Design review of the part built by this model. Coordinates are the model's own, in mm. Face numbers are marked on the shaded views. A direction names the side the tool comes from. Give positions to 0.01 mm unless a question says otherwise; leave off trailing zeros. Write each loop counter-clockwise with the first axis right and the second up, starting at its lowest first coordinate (ties: lowest second). Pieces come first, ordered by that corner, then holes. Notation, with made-up numbers: (-33.75, -26.5) -> (-7.75, -26.5) arc R24 cw to (-7.75, -6.5) -> close; hole circle Ø10 at (-12.75, 47). An arc over 180 degrees is marked (long way). Write each question's results on one line, items separated by ' | '. Start each with the question number.
(1) To check wall thickness, follow probe 1 along Z at (x, y) = (1.5, 10.5); probe 2 along Y at (x, z) = (-5.5, 14.5); probe 3 along Y at (x, z) = (-12, -17.3). State the ranges of each line that lie inside material, in increasing order.
(2) Clearance check with a flat-ended pin moving along its axis: pin 1 (15 mm diameter, centred on x = 3.5, z = -4, fed in from -Y). State where the tip first meets the part, or that it passes through.
(3) Mouldability with a two-part tool opening along Z and no side actions: class the marked faces 3, 4, 5 and 6 as released by +Z, released by -Z, zero draft, split by the parting line, or undercut.
(4) Take a section at D-D (y = 5). State the section outline as (x, z) points, plus the area to 3 significant figures.
(5) Take a section at B-B (z = 0). State the section outline as (x, y) points, plus the area to 3 significant figures.
(6) Take a section at C-C (y = -23.5). State the section outline as (x, z) points, plus the area to 3 significant figures.
(7) For the marked faces 1 and 2, list the 3-axis set-ups (+Z, -Z, +X, -X, +Y, -Y) from which the entire face can be reached by the end or side of a thin tool; tool diameter is ignored.
(8) Take a section at A-A (x = -12). State the section outline as (y, z) points.
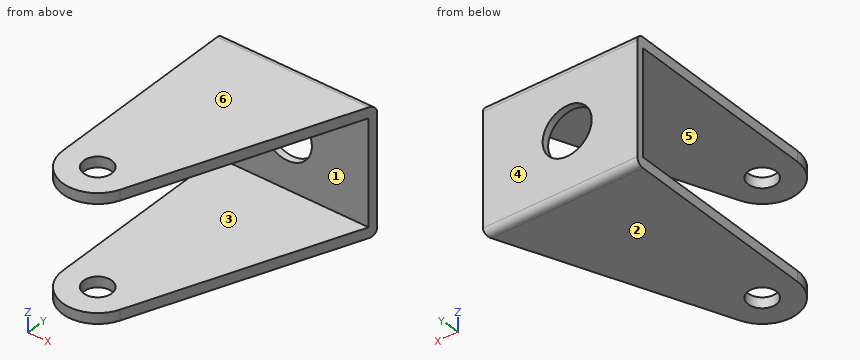
from build123d import *

# Parameters (mm, degrees)
SKETCH_1_R              = 4
EXTRUDE_1_DEPTH         = 18
CUT_EXTRUDE_1_DEPTH     = 15
HOLE_WIZARD_14_0_14_1_D = 14
FILLET_1_R              = 2


with BuildPart() as part:
    # 草图1 → 凸台-拉伸1 (new, symmetric)
    with BuildSketch(Plane.XY):
        with BuildLine():
            Line((-22, 34.943115606), (22, 34.943115606))
            Line((22, 34.943115606), (-2.728161454, -26.261231719))
            ThreePointArc((-2.728161454, -26.261231719), (-13.908089954, -32.331437619), (-22, -22.515165785))
            Line((-22, -22.515165785), (-22, 34.943115606))
        make_face()
        with Locations((-12, -22.515165785)):
            Circle(SKETCH_1_R, mode=Mode.SUBTRACT)
    extrude(amount=EXTRUDE_1_DEPTH, both=True)

    # 草图2 → 切除-拉伸1 (cut, symmetric)
    with BuildSketch(Plane.XY):
        with BuildLine():
            Line((-22, 32.943115606), (21.191947548, 32.943115606))
            Line((21.191947548, 32.943115606), (-2.728161454, -26.261231719))
            ThreePointArc((-2.728161454, -26.261231719), (-13.908089954, -32.331437619), (-22, -22.515165785))
            Line((-22, -22.515165785), (-22, 32.943115606))
        make_face()
    extrude(amount=CUT_EXTRUDE_1_DEPTH, both=True, mode=Mode.SUBTRACT)

    # Ø14.0 (14) 直径孔1 (through all)
    with Locations(Plane(origin=(0, 34.943115606, 0), x_dir=(1, 0, 0), z_dir=(0, 1, 0))):
        with Locations((-2, 0)):
            Hole(HOLE_WIZARD_14_0_14_1_D / 2)

    # 圆角1
    fillet_1_edges = [part.edges().sort_by_distance(p)[0] for p in [
        (0, 34.943115606, 18),
        (0, 34.943115606, -18),
    ]]
    fillet(fillet_1_edges, radius=FILLET_1_R)


solid = part.part
Report:
1) probe 1: -18 to -15, 15 to 18 | probe 2: 32.94 to 34.94 | probe 3: -32.52 to -26.52, -18.52 to 34.46
2) pin 1: y = 32.94
3) face 3: undercut | face 4: zero draft | face 5: undercut | face 6: released by +Z
4) outline: (-22, -18) -> (9.9, -18) -> (9.9, -15) -> (-22, -15) -> close; (-22, 15) -> (9.9, 15) -> (9.9, 18) -> (-22, 18) -> close | area: 191 mm2
5) outline: (-22, 32.94) -> (-9, 32.94) -> (-9, 34.94) -> (-22, 34.94) -> close; (5, 32.94) -> (21.19, 32.94) -> (22, 34.94) -> (5, 34.94) -> close | area: 59.2 mm2
6) outline: (-21.95, -18) -> (-15.88, -18) -> (-15.88, -15) -> (-21.95, -15) -> close; (-21.95, 15) -> (-15.88, 15) -> (-15.88, 18) -> (-21.95, 18) -> close; (-8.12, -18) -> (-1.61, -18) -> (-1.61, -15) -> (-8.12, -15) -> close; (-8.12, 15) -> (-1.61, 15) -> (-1.61, 18) -> (-8.12, 18) -> close | area: 75.5 mm2
7) face 1: +X, -X, -Y | face 2: -Z, +X, -X, +Y, -Y
8) outline: (-32.52, -18) -> (-26.52, -18) -> (-26.52, -15) -> (-32.52, -15) -> close; (-32.52, 15) -> (-26.52, 15) -> (-26.52, 18) -> (-32.52, 18) -> close; (-18.52, -18) -> (32.94, -18) arc R2 ccw to (34.94, -16) -> (34.94, 16) arc R2 ccw to (32.94, 18) -> (-18.52, 18) -> (-18.52, 15) -> (32.94, 15) -> (32.94, -15) -> (-18.52, -15) -> close
